```python
from build123d import *

# Parameters (mm, degrees)
F0_W     = 1900
F0_H     = 1000
F1_DEPTH = 30
F2_R     = 50


with BuildPart() as f1:
    # F0 (on Top) → F1 (new body)
    with BuildSketch(Plane.XY):
        Rectangle(F0_W, F0_H)
    extrude(amount=F1_DEPTH)

    # F2
    f2_edges = [f1.edges().sort_by_distance(p)[0] for p in [
        (-950, -500, 15),
        (-950, 500, 15),
        (950, -500, 15),
        (950, 500, 15),
    ]]
    fillet(f2_edges, radius=F2_R)

    # F6: sweep along a path in F5
    with BuildLine(Plane.XY.offset(30)) as f6_path:
        Line((900, 500), (-900, 500))
        ThreePointArc((-900, 500), (-935.3553390593, 485.3553390593), (-950, 450))
        Line((-950, 450), (-950, -450))
        ThreePointArc((-950, -450), (-935.3553390593, -485.3553390593), (-900, -500))
        Line((-900, -500), (900, -500))
        ThreePointArc((900, -500), (935.3553390593, -485.3553390593), (950, -450))
        Line((950, -450), (950, 450))
        ThreePointArc((950, 450), (935.3553390593, 485.3553390593), (900, 500))
    # F4 (on offset) → F6 (sweep)
    with BuildSketch(Plane.XZ.offset(450)):
        with BuildLine():
            Line((953.3333333333, 30), (950, 30))
            Line((950, 30), (950, 0))
            Line((950, 0), (1000, 0))
            Line((1000, 0), (965.3333333333, 26))
            ThreePointArc((965.3333333333, 26), (959.6578886537, 28.973665961), (953.3333333333, 30))
        make_face()
    sweep(path=f6_path.line)


solid = f1.part
```
Check sheet for the modelled part. Datum: model origin and axes. Units: mm. Round coordinates to 2 decimals unless told otherwise and drop trailing zeros. Write each loop counter-clockwise with the first axis right and the second up, starting at its lowest first coordinate (ties: lowest second). Pieces come first, ordered by that corner, then holes. Notation, with made-up numbers: M 27,46.5 L 72,46.5 A5 ccw 72,51.5 Z; hole C 45,63.25 d4. An arc over 180 degrees is marked long. Write item = value, one per line. Start each with the question number.
1. Section check A-A, the plane z = 7.5. Record the cut outline in (x, y).
2. Section check C-C, the plane y = 141. Record the cut outline in (x, z).
3. Section check B-B, the plane x = -203.5. Record the cut outline in (y, z).
4. Gauge pin test, flat ends, axial feed: pin 1 (10 mm diameter, centred on y = -351.5, z = 26.5, fed in from -X); pin 2 (10 mm diameter, centred on x = 304, z = 6.5, fed in from -Y); pin 3 (10 mm diameter, centred on y = 439, z = 19, fed in from +X). Record the tip position at first contact, or that the pin passes through.
5. Scan lines: line 1 (X direction, y = 270, z = 11); line 2 (X direction, y = 423.5, z = 18.5); line 3 (Y direction, x = 641, z = 21). Record each from-to range of solid material in increasing order. Write a range as [from, to].
Results found:
q1.outline = M -990,-450 A90 ccw -900,-540 L 900,-540 A90 ccw 990,-450 L 990,450 A90 ccw 900,540 L -900,540 A90 ccw -990,450 Z
q2.outline = M -1000,0 L 1000,0 L 965.33,26 A20 ccw 953.33,30 L -953.33,30 A20 ccw -965.33,26 Z
q3.outline = M -550,0 L 550,0 L 515.33,26 A20 ccw 503.33,30 L -503.33,30 A20 ccw -515.33,26 Z
q4.pin_1 = -971.33
q4.pin_2 = -548
q4.pin_3 = 981.33
q5.line_1 = [-985.33, 985.33]
q5.line_2 = [-975.33, 975.33]
q5.line_3 = [-522, 522]
